```python
from build123d import *

# Parameters (mm, degrees)
BOSS_EXTRUDE1_DEPTH  = 3
FILLET1_R            = 5
FILLET2_R            = 5
SKETCH2_W            = 3
SKETCH2_H            = 7
CUT_EXTRUDE1_DEPTH   = 3
LPATTERN1_COUNT      = 3
LPATTERN1_PITCH      = 14
LPATTERN1_COUNT_DIR2 = 2
LPATTERN1_PITCH_DIR2 = 10
CUT_EXTRUDE2_DEPTH   = 3
LPATTERN2_COUNT      = 2
LPATTERN2_PITCH      = 25.5
LPATTERN2_COUNT_DIR2 = 2
LPATTERN2_PITCH_DIR2 = 15.7
FILLET3_R            = 5
FILLET4_R            = 5
FILLET5_R            = 5
FILLET6_R            = 5
FILLET7_R            = 5
FILLET8_R            = 5
CUT_EXTRUDE3_DEPTH   = 3
LPATTERN3_COUNT      = 2
LPATTERN3_PITCH      = 22
SKETCH5_W            = 3
SKETCH5_H            = 7
CUT_EXTRUDE4_DEPTH   = 3
LPATTERN4_COUNT      = 2
LPATTERN4_PITCH      = 14


with BuildPart() as part:
    # Sketch1 → Boss-Extrude1 (new body)
    with BuildSketch(Plane(origin=(0, 0, 0), x_dir=(1, 0, 0), z_dir=(0, 1, 0))):
        Polygon((15, -32.5), (50, -32.5), (50, 32.5), (-50, 32.5), (-50, -32.5), (-15, -32.5), (-15, 2.5), (15, 2.5), align=None)
    extrude(amount=BOSS_EXTRUDE1_DEPTH)

    # Fillet1
    fillet1_edges = [part.edges().sort_by_distance(p)[0] for p in [
        (-15, 1.5, -2.5),
    ]]
    fillet(fillet1_edges, radius=FILLET1_R)

    # Fillet2
    fillet2_edges = [part.edges().sort_by_distance(p)[0] for p in [
        (15, 1.5, -2.5),
    ]]
    fillet(fillet2_edges, radius=FILLET2_R)

    # Sketch2 → Cut-Extrude1 (cut)
    with BuildSketch(Plane(origin=(0, 3, 0), x_dir=(1, 0, 0), z_dir=(0, 1, 0))):
        with Locations((-20.5, 3)):
            Rectangle(SKETCH2_W, SKETCH2_H)
    cut_extrude1 = extrude(amount=-CUT_EXTRUDE1_DEPTH, mode=Mode.SUBTRACT)

    # LPattern1: Cut-Extrude1 3 × 2
    with Locations(*[(-j * LPATTERN1_PITCH_DIR2, 0, i * LPATTERN1_PITCH) for i in range(LPATTERN1_COUNT) for j in range(LPATTERN1_COUNT_DIR2) if (i, j) != (0, 0)]):
        add(cut_extrude1, mode=Mode.SUBTRACT)

    # Sketch3 → Cut-Extrude2 (cut)
    with BuildSketch(Plane(origin=(0, 3, 0), x_dir=(1, 0, 0), z_dir=(0, 1, 0))):
        Polygon((-13.55, 28.5), (-11.95, 28.5), (-11.95, 26.9), (-10.35, 26.9), (-10.35, 25.3), (-11.95, 25.3), (-11.95, 23.7), (-13.55, 23.7), (-13.55, 25.3), (-15.15, 25.3), (-15.15, 26.9), (-13.55, 26.9), align=None)
    cut_extrude2 = extrude(amount=-CUT_EXTRUDE2_DEPTH, mode=Mode.SUBTRACT)

    # LPattern2: Cut-Extrude2 2 × 2
    with Locations(*[(i * LPATTERN2_PITCH, 0, j * LPATTERN2_PITCH_DIR2) for i in range(LPATTERN2_COUNT) for j in range(LPATTERN2_COUNT_DIR2) if (i, j) != (0, 0)]):
        add(cut_extrude2, mode=Mode.SUBTRACT)

    # Fillet3
    fillet3_edges = [part.edges().sort_by_distance(p)[0] for p in [
        (-50, 1.5, -32.5),
    ]]
    fillet(fillet3_edges, radius=FILLET3_R)

    # Fillet4
    fillet4_edges = [part.edges().sort_by_distance(p)[0] for p in [
        (50, 1.5, -32.5),
    ]]
    fillet(fillet4_edges, radius=FILLET4_R)

    # Fillet5
    fillet5_edges = [part.edges().sort_by_distance(p)[0] for p in [
        (-50, 1.5, 32.5),
    ]]
    fillet(fillet5_edges, radius=FILLET5_R)

    # Fillet6
    fillet6_edges = [part.edges().sort_by_distance(p)[0] for p in [
        (50, 1.5, 32.5),
    ]]
    fillet(fillet6_edges, radius=FILLET6_R)

    # Fillet7
    fillet7_edges = [part.edges().sort_by_distance(p)[0] for p in [
        (15, 1.5, 32.5),
    ]]
    fillet(fillet7_edges, radius=FILLET7_R)

    # Fillet8
    fillet8_edges = [part.edges().sort_by_distance(p)[0] for p in [
        (-15, 1.5, 32.5),
    ]]
    fillet(fillet8_edges, radius=FILLET8_R)

    # Sketch4 → Cut-Extrude3 (cut)
    with BuildSketch(Plane(origin=(0, 3, 0), x_dir=(1, 0, 0), z_dir=(0, 1, 0))):
        with BuildLine():
            Line((31, 25.5), (31, 15.5))
            ThreePointArc((31, 15.5), (28, 12.5), (25, 15.5))
            Line((25, 15.5), (25, 25.5))
            ThreePointArc((25, 25.5), (28, 28.5), (31, 25.5))
        make_face()
    cut_extrude3 = extrude(amount=-CUT_EXTRUDE3_DEPTH, mode=Mode.SUBTRACT)

    # LPattern3: Cut-Extrude3 ×2
    with Locations(*[(0, 0, i * LPATTERN3_PITCH) for i in range(1, LPATTERN3_COUNT)]):
        add(cut_extrude3, mode=Mode.SUBTRACT)

    # Sketch5 → Cut-Extrude4 (cut)
    with BuildSketch(Plane(origin=(0, 3, 0), x_dir=(1, 0, 0), z_dir=(0, 1, 0))):
        with Locations((-45.5, -4)):
            Rectangle(SKETCH5_W, SKETCH5_H)
    cut_extrude4 = extrude(amount=-CUT_EXTRUDE4_DEPTH, mode=Mode.SUBTRACT)

    # LPattern4: Cut-Extrude4 ×2
    with Locations(*[(0, 0, i * LPATTERN4_PITCH) for i in range(1, LPATTERN4_COUNT)]):
        add(cut_extrude4, mode=Mode.SUBTRACT)


solid = part.part
```
Input: part model. Units: mm. Frame: model coordinates. A direction names the side the tool comes from. Round coordinates to 2 decimals unless told otherwise and drop trailing zeros. Loops run counter-clockwise (first coordinate to the right, second up) from the corner with the lowest first, then second, coordinate; pieces in that order, holes last. Notation, with made-up numbers: (-31.75, 60) -> (-5.75, 60) arc R17 cw to (-5.75, 76) -> close; hole circle Ø8 at (-15.75, 54.5). An arc over 180 degrees is marked (long way). Write each question's results on one line, items separated by ' | '.
1. Section B-B (x = 29). Return loops of the section in (y, z).
Geometry results:
outline: (0, -32.5) -> (3, -32.5) -> (3, -28.33) -> (0, -28.33) -> close; (0, -12.67) -> (3, -12.67) -> (3, -6.33) -> (0, -6.33) -> close; (0, 9.33) -> (3, 9.33) -> (3, 32.5) -> (0, 32.5) -> close
2. First-contact query: P1, Ø1, axis at x = -0.5, y = 1.5, coming from the +Z side; P2, Ø1.5, axis at x = -45.5, y = 2, coming from the -Z side; P3, Ø0.5, axis at x = 13, y = 1, coming from the +Z side. Flat tips, straight axial feed; report the tip coordinate or a pass-through.
Geometry results:
P1: z = -2.5 | P2: z = -32.5 | P3: z = -1.3
3. Set-up query: faces 4 (the face through (15, 1, 15)), 5 (the face through (-47, 2, 18)). Return all of +Z, -Z, +X, -X, +Y, -Y with unobstructed straight access to the full face (end or side cutting, diameter ignored); none if empty.
Geometry results:
face 4: +Z, +Y, -Y | face 5: +Y, -Y
4. Ray query, line 1 (Z direction, x = -29.5, y = 2.3); line 2 (X direction, y = 2.7, z = 10.5); line 3 (X direction, y = 1.8, z = 18). Return the intervals inside material, ascending. Write a range as from..to.
Geometry results:
line 1: -32.5..-6.5, 0.5..7.5, 14.5..21.5, 28.5..32.5 | line 2: -50..-32, -29..-22, -19..-15, 15..50 | line 3: -50..-47, -44..-15, 15..50
5. Mould query, pull axis X, two halves, no side actions, for faces 1 (the face through (-50, 1, 0)), 2 (the face through (-1, 3, -8)), 3 (the face through (-47, 2, 4)). Classes: +X half, -X half, draft (parallel to the pull), parting line (faces both ways), or undercut.
Geometry results:
face 1: -X half | face 2: draft | face 3: undercut
6. Section C-C (y = 0.75). State how many separate pieces and enclosed holes the cut face has, and give its area (3 significant figures).
Geometry results:
separate pieces: 1 | enclosed holes: 14 | area: 5,030 mm2
7. Section A-A (z = 11.5). Return loops of the section in (x, y), and give its area (3 significant figures).
Geometry results:
outline: (-50, 0) -> (-32, 0) -> (-32, 3) -> (-50, 3) -> close; (-29, 0) -> (-22, 0) -> (-22, 3) -> (-29, 3) -> close; (-19, 0) -> (-15, 0) -> (-15, 3) -> (-19, 3) -> close; (15, 0) -> (50, 0) -> (50, 3) -> (15, 3) -> close | area: 192 mm2
